from build123d import *

# Parameters (mm, degrees)
MODEL_R                 = 1.5
SALIENTE_EXTRUIR1_DEPTH = 3


with BuildPart() as part:
    # Model → Saliente-Extruir1 (new body)
    with BuildSketch(Plane.XY):
        with BuildLine():
            Line((174.227054575, 190.675884941), (192.227054575, 190.675884941))
            Line((192.227054575, 190.675884941), (192.227054575, 213.178720063))
            ThreePointArc((192.227054575, 213.178720063), (190.90903509, 216.360700578), (187.727054575, 217.678720063))
            Line((187.727054575, 217.678720063), (178.727054575, 217.678720063))
            ThreePointArc((178.727054575, 217.678720063), (175.545074059, 216.360700578), (174.227054575, 213.178720063))
            Line((174.227054575, 213.178720063), (174.227054575, 190.675884941))
        make_face()
        with Locations((183.227054575, 199.678720063)):
            Circle(MODEL_R, mode=Mode.SUBTRACT)
        with Locations((183.227054575, 208.632069818)):
            Circle(MODEL_R, mode=Mode.SUBTRACT)
        with Locations((187.727054575, 204.178720063)):
            Circle(MODEL_R, mode=Mode.SUBTRACT)
        with Locations((178.727054575, 204.178720063)):
            Circle(MODEL_R, mode=Mode.SUBTRACT)
        with Locations((187.727054575, 213.178720063)):
            Circle(MODEL_R, mode=Mode.SUBTRACT)
        with Locations((178.727054575, 213.178720063)):
            Circle(MODEL_R, mode=Mode.SUBTRACT)
        with BuildLine():
            Line((190.227058417, 193.553720063), (185.227058417, 193.553720063))
            ThreePointArc((185.227058417, 193.553720063), (184.696728331, 193.773389977), (184.477058417, 194.303720063))
            Line((184.477058417, 194.303720063), (184.477058417, 196.053720063))
            ThreePointArc((184.477058417, 196.053720063), (184.696728331, 196.584050149), (185.227058417, 196.803720063))
            Line((185.227058417, 196.803720063), (190.227058417, 196.803720063))
            ThreePointArc((190.227058417, 196.803720063), (190.757388503, 196.584050149), (190.977058417, 196.053720063))
            Line((190.977058417, 196.053720063), (190.977058417, 194.303720063))
            ThreePointArc((190.977058417, 194.303720063), (190.757388503, 193.773389977), (190.227058417, 193.553720063))
        make_face(mode=Mode.SUBTRACT)
        with BuildLine():
            Line((181.227058417, 193.553720063), (176.227058417, 193.553720063))
            ThreePointArc((176.227058417, 193.553720063), (175.696728331, 193.773389977), (175.477058417, 194.303720063))
            Line((175.477058417, 194.303720063), (175.477058417, 196.053720063))
            ThreePointArc((175.477058417, 196.053720063), (175.696728331, 196.584050149), (176.227058417, 196.803720063))
            Line((176.227058417, 196.803720063), (181.227058417, 196.803720063))
            ThreePointArc((181.227058417, 196.803720063), (181.757388503, 196.584050149), (181.977058417, 196.053720063))
            Line((181.977058417, 196.053720063), (181.977058417, 194.303720063))
            ThreePointArc((181.977058417, 194.303720063), (181.757388503, 193.773389977), (181.227058417, 193.553720063))
        make_face(mode=Mode.SUBTRACT)
    extrude(amount=SALIENTE_EXTRUIR1_DEPTH)


solid = part.part
Geometry: final body of the model. Coordinates: model frame, mm. A direction names the side the tool comes from. Give positions to 0.01 mm unless a question says otherwise; leave off trailing zeros. Write each loop counter-clockwise with the first axis right and the second up, starting at its lowest first coordinate (ties: lowest second). Pieces come first, ordered by that corner, then holes. Notation, with made-up numbers: (5, 50.5) -> (25, 50.5) arc R22 ccw to (25, 73.5) -> close; hole circle Ø5 at (5.25, -31.5). An arc over 180 degrees is marked (long way). Answer in a Markdown table with one row per item.
(1) Section query A-A on x = 185.5. Return loops of the section in (y, z).
Answers below:
| item | result |
|---|---|
| outline | (190.68, 0) -> (193.55, 0) -> (193.55, 3) -> (190.68, 3) -> close; (196.8, 0) -> (217.68, 0) -> (217.68, 3) -> (196.8, 3) -> close |
(2) Section query C-C on z = 1.9. State how many separate pieces and enclosed holes the cut face has, then the cut area to 3 significant figures.
Answers below:
| item | result |
|---|---|
| separate pieces | 1 |
| enclosed holes | 8 |
| area | 394 mm^2 |
(3) Section query B-B on y = 194.75. Return loops of the section in (x, z), then the cut area to 3 significant figures.
Answers below:
| item | result |
|---|---|
| outline | (174.23, 0) -> (175.48, 0) -> (175.48, 3) -> (174.23, 3) -> close; (181.98, 0) -> (184.48, 0) -> (184.48, 3) -> (181.98, 3) -> close; (190.98, 0) -> (192.23, 0) -> (192.23, 3) -> (190.98, 3) -> close |
| area | 15.0 mm^2 |
(4) Ray query, line 1 along Y through (x, z) = (185.25, 2.2); line 2 along X through (y, z) = (214, 1.95); line 3 along Y through (x, z) = (186.75, 2.7). Return the intervals inside material, ascending. Write a range as [from, to].
Answers below:
| item | result |
|---|---|
| line 1 | [190.68, 193.55], [196.8, 217.68] |
| line 2 | [174.3, 177.47], [179.98, 186.47], [188.98, 192.15] |
| line 3 | [190.68, 193.55], [196.8, 203.04], [205.32, 212.04], [214.32, 217.68] |
(5) Section query D-D on y = 200.5. Return loops of the section in (x, z), then the cut area to 3 significant figures.
Answers below:
| item | result |
|---|---|
| outline | (174.23, 0) -> (181.97, 0) -> (181.97, 3) -> (174.23, 3) -> close; (184.48, 0) -> (192.23, 0) -> (192.23, 3) -> (184.48, 3) -> close |
| area | 46.5 mm^2 |
(6) Set-up query: faces 4 (the cylindrical face through (190.94, 216.33, 1.48)), 5 (the flat face through (179, 196.804, 1)). Return all of +Z, -Z, +X, -X, +Y, -Y with unobstructed straight access to the full face (end or side cutting, diameter ignored); none if empty.
Answers below:
| item | result |
|---|---|
| face 4 | +Z, -Z, +X, +Y |
| face 5 | +Z, -Z |
(7) Draft query along X for faces 1 (the cylindrical face through (175.58, 216.395, 1.479)), 2 (the cylindrical face through (188.533, 214.444, 1.479)), 3 (the flat face through (183, 204, 0)). Return one class per face: +X half, -X half, draft (parallel to the pull), parting line (faces both ways), or undercut.
Answers below:
| item | result |
|---|---|
| face 1 | -X half |
| face 2 | undercut |
| face 3 | draft |
